Print and shaded views of the part. All mm, measured from the part's lowest x, y and z. A direction names the side the tool comes from. Round coordinates to 2 decimals unless told otherwise and drop trailing zeros. Write each loop counter-clockwise with the first axis right and the second up, starting at its lowest first coordinate (ties: lowest second). Pieces come first, ordered by that corner, then holes. Notation, with made-up numbers: (-29, 41.5) - (14, 41.5) arc R30 ccw to (14, 77.5) - close; hole circle Ø6 at (48, 65). An arc over 180 degrees is marked (long way). One line per item, written item: value.
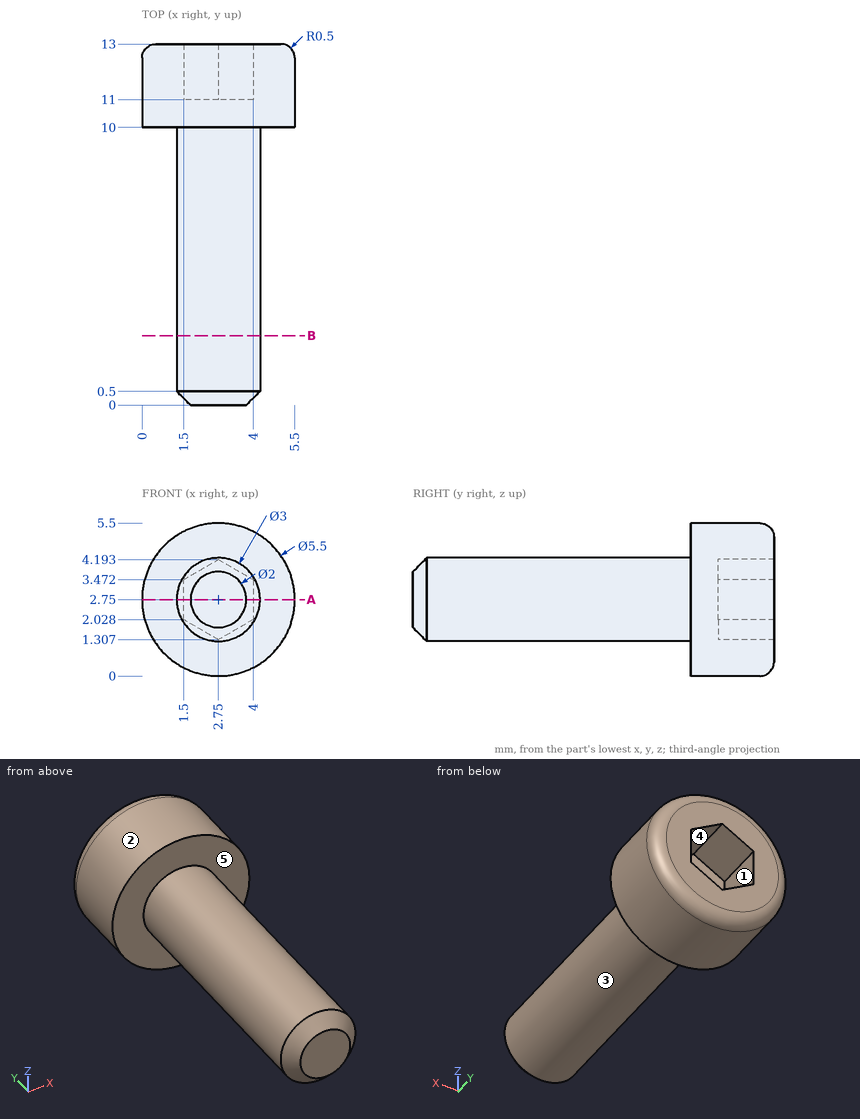
1. Wall check: probe 1 along Y at (x, z) = (0.85, 3.15); probe 2 along Y at (x, z) = (2.2, 3.3); probe 3 along Z at (x, y) = (3.45, 12.25). Give the ranges that are in metal, low to high. Write a range as [from, to].
Report:
probe 1: [10, 13]
probe 2: [0, 11]
probe 3: [0.09, 1.71], [3.79, 5.41]
2. Drop flat-ended pins along their axis: pin 1 (3 mm diameter, centred on y = 6.5, z = 0.5, fed in from +X); pin 2 (1.5 mm diameter, centred on x = 1, y = 3.5, fed in from -Z); pin 3 (1 mm diameter, centred on x = 1.5, z = 1, fed in from -Y). Give the stop position or say it passes through.
Report:
pin 1: x = 4.05
pin 2: z = 1.63
pin 3: y = 10
3. Band-saw the part on B-B on y = 2.5. Write the cut outline in (x, z).
Report:
outline: circle Ø3 at (2.75, 2.75)
4. Mould opens along Z. For the marked faces 3, 4 and 5 say: released by +Z, released by -Z, zero draft, split by the parting line, or undercut.
Report:
face 3: split by the parting line
face 4: undercut
face 5: zero draft
5. Band-saw the part on A-A on z = 2.75. Write the cut outline in (x, y).
Report:
outline: (0, 10) - (1.25, 10) - (1.25, 0.5) - (1.75, 0) - (3.75, 0) - (4.25, 0.5) - (4.25, 10) - (5.5, 10) - (5.5, 12.5) arc R0.5 ccw to (5, 13) - (4, 13) - (4, 11) - (1.5, 11) - (1.5, 13) - (0.5, 13) arc R0.5 ccw to (0, 12.5) - close
6. Tool access for the marked faces 1 and 2: list every direction of +Z, -Z, +X, -X, +Y, -Y with a clear straight run to the whole face (end or side of a thin tool).
Report:
face 1: +Y
face 2: +Y, -Y
